Geometry check sheet. Reference: the model listing, model coordinates, mm. Give positions to 0.01 mm unless a question says otherwise; leave off trailing zeros. Loops run counter-clockwise (first coordinate to the right, second up) from the corner with the lowest first, then second, coordinate; pieces in that order, holes last. Notation, with made-up numbers: (38, 74.5) - (59, 74.5) arc R15 ccw to (59, 80.5) - close; hole circle Ø5 at (61.25, 28.25). An arc over 180 degrees is marked (long way). One line per question, with ' | ' between items. Start each with the question number.
Autodesk Inventor part; units mm, degrees
ref_plane "YZ Plane" through (0, 0, 0) normal (1, 0, 0) x (0, 1, 0)
ref_plane "XZ Plane" through (0, 0, 0) normal (0, 1, 0) x (-1, 0, 0)
ref_plane "XY Plane" through (0, 0, 0) normal (0, 0, 1) x (1, 0, 0)
sketch "Sketch1" plane through (0, 0, 0) normal (0, 0, 1) x (1, 0, 0)
  line L0 (0, 0) -> (41.5, 0)
  line L1 (41.5, 0) -> (41.5, 15)
  line L2 (41.5, 15) -> (0, 15)
  line L3 (0, 15) -> (0, 0)
  line L4 (0, 7.5) -> (41.5, 7.5) construction
  line L5 (20.75, 15) -> (20.75, 0) construction
  circle A0 centre (20.75, 7.5) radius 16 construction
  circle A1 centre (4.75, 7.5) radius 2.35
  circle A2 centre (36.75, 7.5) radius 2.35
  dimension "d0" = 41.5
  dimension "d1" = 15
  dimension "d2" = 32
  dimension "d3" = 4.7
  dimension "d4" = 4.7
extrude "Extrusion1" add sketch "Sketch1" along normal blind 3
chamfer "Chamfer1" distance 3 angle 45 4 edges at (0, 15, 1.5) (41.5, 15, 1.5) (41.5, 0, 1.5) (0, 0, 1.5)
fillet "Fillet1" radius 0.5 8 edges at (1.5, 1.5, 3) (20.75, 0, 3) (40, 1.5, 3) (41.5, 7.5, 3) (40, 13.5, 3) (20.75, 15, 3) (1.5, 13.5, 3) (0, 7.5, 3)
properties part number "MagneticLimitBaseSpacer3milTall"
(1) Section check B-B, the plane y = 7.5. Record the boundary of the cut face in (x, z).
(2) Section check A-A, the plane x = 4.75. Record the boundary of the cut face in (y, z), and give its area (3 significant figures).
(3) Material ranges on line 1 (Y direction, x = 36.75, z = 2.05); line 2 (X direction, y = 5.5, z = 1.45); line 3 (Y direction, x = 36, z = 2.35), recorded low to high.
(4) Section check C-C, the plane z = 1.55. Record the boundary of the cut face in (x, y).
(5) Mould release check, pull along X, two halves, no side actions. Record for faces 1 (the face through (5.834, 9.585, 1.479)), 2 (the face through (1.63, 1.59, 2.86)), 3 (the face through (39.92, 13.38, 2.85)): pulls with the +X half, pulls with the -X half, needs draft (parallel to the pull), parting line crosses it, or undercut.
(6) Depth check by flat-ended pin: pin 1 Ø3 at (x, y) = (36.75, 7.5) entering from -Z; pin 2 Ø1.5 at (y, z) = (9.5, 0.5) entering from -X. Enter the tip coordinate at first touch or a pass-through.
Numbers:
1) outline: (0, 0) - (2.4, 0) - (2.4, 3) - (0.5, 3) arc R0.5 ccw to (0, 2.5) - close; (7.1, 0) - (34.4, 0) - (34.4, 3) - (7.1, 3) - close; (39.1, 0) - (41.5, 0) - (41.5, 2.5) arc R0.5 ccw to (41, 3) - (39.1, 3) - close
2) outline: (0, 0) - (5.15, 0) - (5.15, 3) - (0.5, 3) arc R0.5 ccw to (0, 2.5) - close; (9.85, 0) - (15, 0) - (15, 2.5) arc R0.5 ccw to (14.5, 3) - (9.85, 3) - close | area: 30.8 mm^2
3) line 1: 0 to 5.15, 9.85 to 15 | line 2: 0 to 3.52, 5.98 to 35.52, 37.98 to 41.5 | line 3: 0 to 5.27, 9.73 to 15
4) outline: (0, 3) - (3, 0) - (38.5, 0) - (41.5, 3) - (41.5, 12) - (38.5, 15) - (3, 15) - (0, 12) - close; hole circle Ø4.7 at (4.75, 7.5); hole circle Ø4.7 at (36.75, 7.5)
5) face 1: undercut | face 2: pulls with the -X half | face 3: pulls with the +X half
6) pin 1: through | pin 2: x = 0
